Here's how the part is built. I have some questions about the finished solid (model axes, mm). Coordinates: 2 decimals unless noted, no trailing zeros. Write each loop counter-clockwise with the first axis right and the second up, starting at its lowest first coordinate (ties: lowest second). Pieces come first, ordered by that corner, then holes. Notation, with made-up numbers: (-26.75, 45.25) - (-1.75, 45.25) arc R24 cw to (-1.75, 78.25) - close; hole circle Ø6 at (-28.75, 22). An arc over 180 degrees is marked (long way). Answer in a Markdown table with one row per item. Add a question column.
Item 1: Imagine slicing it at B-B (x = 13). Please give me the cut outline in (y, z), plus the area to 3 significant figures.
Item 2: If I drill on probe 1 along Y at (x, z) = (0, -1.55); probe 2 along X at (y, z) = (142, -1.1); probe 3 along Y at (x, z) = (4, -1.9), over which ranges is the centre line in solid material (lowest first)? Write a range as from..to.
Item 3: I'm going to push flat-ended pins straight in: pin 1 (0.8 mm diameter, centred on y = 140.5, z = -1.5, fed in from -X); pin 2 (1.2 mm diameter, centred on y = 143, z = -1.5, fed in from +X); pin 3 (1.2 mm diameter, centred on x = -5, z = -2, fed in from +Y); pin 4 (1.6 mm diameter, centred on x = 0, y = 146.66, fed in from +Z). Where does each tip first touch, or does it pass through?
Item 4: Imagine slicing it at A-A (z = -0.5). Please give me the cut outline in (x, y).
Item 5: Imagine slicing it at C-C (y = 29.5). Please give me the cut outline in (x, z), plus the area to 3 significant figures.
from build123d import *

# Parameters (mm, degrees)
BASE_FLANGE1_DEPTH = 2.5
SKETCH8_R          = 1
CUT_EXTRUDE1_DEPTH = 10


# Sheet-metal steps are written as plain solids
with BuildPart() as part:
    # Sketch1 → Base-Flange1 (new body)
    with BuildSketch(Plane.XY):
        Polygon((-31.5, 0), (31.5, 0), (6.169112777, 130), (2.5, 130), (2.5, 150), (-2.5, 150), (-2.5, 130), (-6.169112777, 130), align=None)
    extrude(amount=-BASE_FLANGE1_DEPTH)

    # Sketch8 → Cut-Extrude1 (cut)
    with BuildSketch(Plane.XY):
        with Locations((0, 146.661825485)):
            Circle(SKETCH8_R)
    extrude(amount=-CUT_EXTRUDE1_DEPTH, mode=Mode.SUBTRACT)


solid = part.part
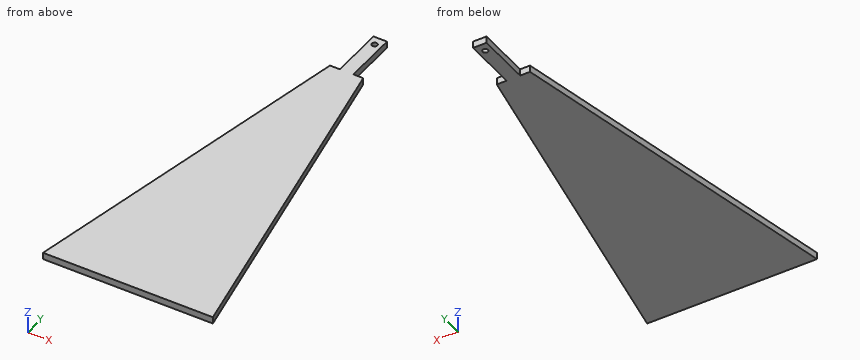
Here are the results:
| question | item | result |
|---|---|---|
| 1 | outline | (0, -2.5) - (94.94, -2.5) - (94.94, 0) - (0, 0) - close |
| 1 | area | 237 mm2 |
| 2 | probe 1 | y = 0..145.66, 147.66..150 |
| 2 | probe 2 | x = -2.5..2.5 |
| 2 | probe 3 | y = 0..130 |
| 3 | pin 1 | stops at x = -2.5 |
| 3 | pin 2 | stops at x = 2.5 |
| 3 | pin 3 | stops at y = 130 |
| 3 | pin 4 | passes through |
| 4 | outline | (-31.5, 0) - (31.5, 0) - (6.17, 130) - (2.5, 130) - (2.5, 150) - (-2.5, 150) - (-2.5, 130) - (-6.17, 130) - close; hole circle Ø2 at (0, 146.66) |
| 5 | outline | (-25.75, -2.5) - (25.75, -2.5) - (25.75, 0) - (-25.75, 0) - close |
| 5 | area | 129 mm2 |
